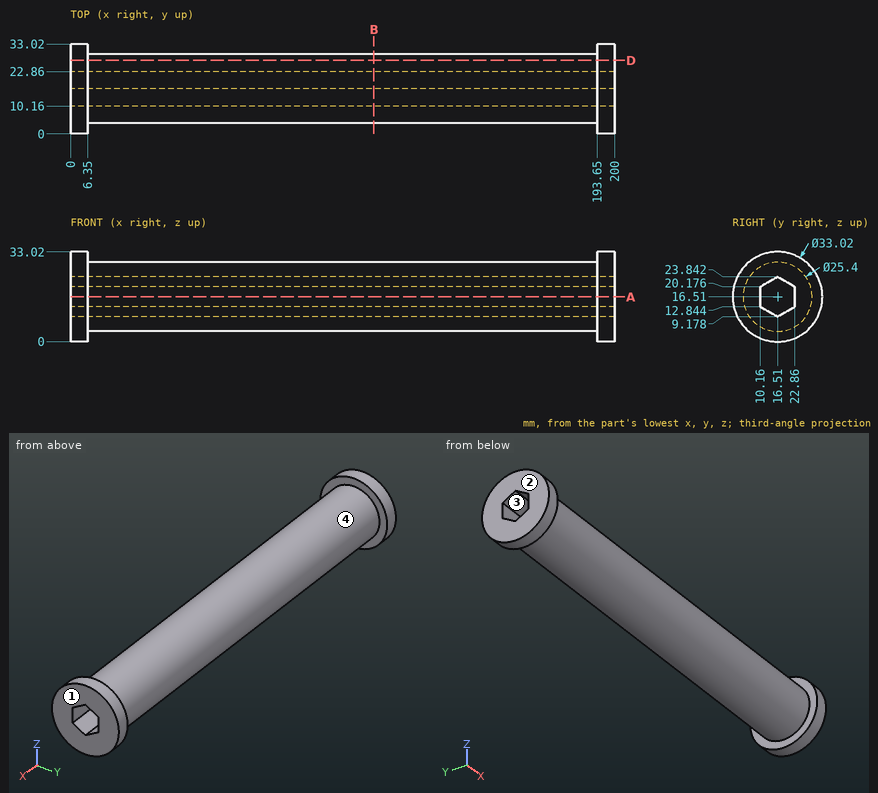
Geometry: see drawing. Coordinates: mm, zero at the bounding-box minimum. Round coordinates to 2 decimals unless told otherwise and drop trailing zeros. Write each loop counter-clockwise with the first axis right and the second up, starting at its lowest first coordinate (ties: lowest second). Pieces come first, ordered by that corner, then holes.
1) Contact query for flat-ended pins moving along their axis: P1, Ø10, axis at y = 4.5, z = 7, coming from the -X side; P2, Ø2, axis at x = 117.5, z = 27, coming from the +Y side; P3, Ø2, axis at x = 105.5, z = 18, coming from the +Y side; P4, Ø6, axis at x = 121.5, z = 16.5, coming from the -Y side. Output: stop coordinate, or through.
2) Draft query along X for the marked faces 1, 2, 3 and 4. Return one class per face: pulls with the +X half, pulls with the -X half, needs draft (parallel to the pull), parting line crosses it, or undercut.
3) Cut plane A-A (z = 16.51). Return the cut outline in (x, y).
4) Cut plane B-B (x = 111.5). Return the cut outline in (y, z).
5) Ray query, L1, parallel to X at y = 19, z = 29; L2, parallel to Z at x = 110.5, y = 20; L3, parallel to Y at x = 159.5, z = 19. Return the intervals inside material, ascending.
6) Cut plane D-D (y = 27). Return the cut outline in (x, z).
Geometry says:
1. P1: stops at x = 0
1. P2: stops at y = 24.95
1. P3: stops at y = 29.2
1. P4: stops at y = 3.81
2. face 1: pulls with the +X half
2. face 2: pulls with the -X half
2. face 3: needs draft
2. face 4: undercut
3. outline: (0, 0) - (6.35, 0) - (6.35, 3.81) - (193.65, 3.81) - (193.65, 0) - (200, 0) - (200, 10.16) - (0, 10.16) - close; (0, 22.86) - (200, 22.86) - (200, 33.02) - (193.65, 33.02) - (193.65, 29.21) - (6.35, 29.21) - (6.35, 33.02) - (0, 33.02) - close
4. outline: circle Ø25.4 at (16.51, 16.51); hole (10.16, 12.84) - (16.51, 9.18) - (22.86, 12.84) - (22.86, 20.18) - (16.51, 23.84) - (10.16, 20.18) - close
5. L1: x = 0 to 6.35, 193.65 to 200
5. L2: z = 4.3 to 11.19, 21.83 to 28.72
5. L3: y = 4.06 to 10.16, 22.86 to 28.96
6. outline: (0, 3.76) - (6.35, 3.76) - (6.35, 9.35) - (193.65, 9.35) - (193.65, 3.76) - (200, 3.76) - (200, 29.26) - (193.65, 29.26) - (193.65, 23.67) - (6.35, 23.67) - (6.35, 29.26) - (0, 29.26) - close
